Here's how the part is built. I have some questions about the finished solid (model axes, mm). Face numbers are marked on the shaded views. A direction names the side the tool comes from. Round coordinates to 2 decimals unless told otherwise and drop trailing zeros. Write each loop counter-clockwise with the first axis right and the second up, starting at its lowest first coordinate (ties: lowest second). Pieces come first, ordered by that corner, then holes. Notation, with made-up numbers: (40.25, 14) -> (57.25, 14) arc R28 ccw to (57.25, 45) -> close; hole circle Ø8 at (-3.75, 10). An arc over 180 degrees is marked (long way). Put each result on its own line as item: value. Start each with the question number.
1) Will these pins go through, and if not, where does the flat tip stop? P1, Ø1, axis at y = -4.5, z = 21.5, coming from the +X side; P2, Ø19, axis at x = -3.5, z = 16.5, coming from the +Y side; P3, Ø3.5, axis at x = -18.5, y = 18, coming from the -Z side; P4, Ø3.5, axis at y = 19, z = 92.3, coming from the -X side.
2) I want a section at B-B, the plane x = -5. List the corners of the cut face in (y, z) for me, then the cut area to 3 significant figures.
3) Which directions (+Z, -Z, +X, -X, +Y, -Y) give clear straight access to the entire face, cutting with the end or side of a thin tool? Please do the marked faces 1, 2, 3, 4 and 5.
4) If I drill on line 1 along Z through (x, y) = (-18.25, 19) (3 decimals); line 2 along Y through (x, z) = (-18, 92); line 3 along X through (y, z) = (-23, 44), over which ranges is the centre line in solid material (lowest first)? Write a range as [from, to].
5) I want a section at A-A, the plane y = -19. List the corners of the cut face in (x, z) for me (3 decimals).
6) I want a section at C-C, the plane z = 26. List the corners of the cut face in (x, y) for me, then the cut area to 3 significant figures.
7) I want a section at D-D, the plane y = -1. List the corners of the cut face in (x, z) for me.
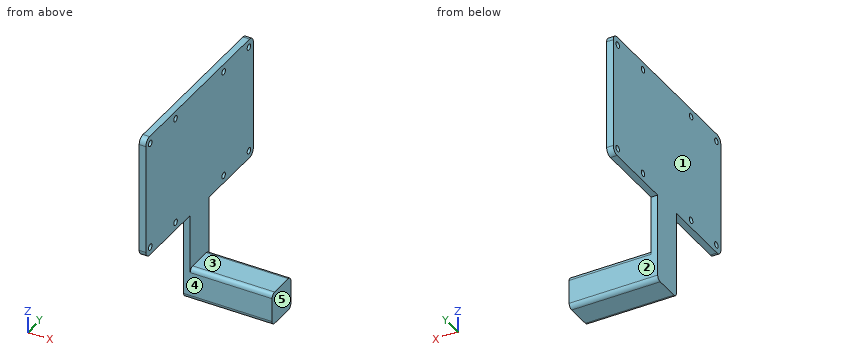
from build123d import *

# Parameters (mm, degrees)
SKETCH1_W           = 40
SKETCH1_H           = 14.8
BOSS_EXTRUDE1_DEPTH = 14.8
SKETCH3_W           = 3
SKETCH3_H           = 14.8
BOSS_EXTRUDE3_DEPTH = 25
SKETCH5_W           = 3
SKETCH5_H           = 85
BOSS_EXTRUDE4_DEPTH = 56
SKETCH6_R           = 1.375
CUT_EXTRUDE1_DEPTH  = 5
FILLET2_R           = 3
FILLET3_R           = 2


with BuildPart() as part:
    # Sketch1 → Boss-Extrude1 (new body)
    with BuildSketch(Plane.XY):
        Rectangle(SKETCH1_W, SKETCH1_H)
    extrude(amount=BOSS_EXTRUDE1_DEPTH)

    # Sketch3 → Boss-Extrude3 (add)
    with BuildSketch(Plane.XY.offset(14.8)):
        with Locations((-18.5, 0)):
            Rectangle(SKETCH3_W, SKETCH3_H)
    extrude(amount=BOSS_EXTRUDE3_DEPTH)

    # Sketch5 → Boss-Extrude4 (add)
    with BuildSketch(Plane.XY.offset(39.8)):
        with Locations((-18.5, 0)):
            Rectangle(SKETCH5_W, SKETCH5_H)
    extrude(amount=BOSS_EXTRUDE4_DEPTH)

    # Sketch6 → Cut-Extrude1 (cut)
    with BuildSketch(Plane(origin=(-17, 0, 0), x_dir=(0, 0, -1), z_dir=(1, 0, 0))):
        with Locations((-92.3, 39)):
            Circle(SKETCH6_R)
        with Locations((-43.3, 39)):
            Circle(SKETCH6_R)
        with Locations((-43.3, -19)):
            Circle(SKETCH6_R)
        with Locations((-92.3, -19)):
            Circle(SKETCH6_R)
    cut_extrude1 = extrude(amount=-CUT_EXTRUDE1_DEPTH, mode=Mode.SUBTRACT)

    # Fillet2
    fillet2_edges = [part.edges().sort_by_distance(p)[0] for p in [
        (-18.5, -42.5, 39.8),
        (-18.5, 42.5, 39.8),
        (-18.5, -42.5, 95.8),
        (-18.5, 42.5, 95.8),
    ]]
    fillet(fillet2_edges, radius=FILLET2_R)

    # Mirror1: Cut-Extrude1 across plane
    add(cut_extrude1.mirror(Plane.ZX), mode=Mode.SUBTRACT)

    # Fillet3
    fillet3_edges = [part.edges().sort_by_distance(p)[0] for p in [
        (1.5, 7.4, 14.8),
        (1.5, -7.4, 14.8),
        (0, 7.4, 0),
        (0, -7.4, 0),
    ]]
    fillet(fillet3_edges, radius=FILLET3_R)


solid = part.part
Findings:
1. P1: stops at x = -17
1. P2: stops at y = 7.4
1. P3: stops at z = 39.8
1. P4: stops at x = -20
2. outline: (-7.4, 2) arc R2 ccw to (-5.4, 0) -> (5.4, 0) arc R2 ccw to (7.4, 2) -> (7.4, 12.8) arc R2 ccw to (5.4, 14.8) -> (-5.4, 14.8) arc R2 ccw to (-7.4, 12.8) -> close
2. area: 216 mm2
3. face 1: +Z, -Z, -X, +Y, -Y
3. face 2: -Z, +X, -X, +Y
3. face 3: +Z, +X, +Y, -Y
3. face 4: -Z, +X, -X, -Y
3. face 5: +Z, -Z, +X, +Y, -Y
4. line 1: z = [39.8, 41.925], [44.675, 90.925], [93.675, 95.8]
4. line 2: y = [-42.5, -40.34], [-37.66, -20.34], [-17.66, 17.66], [20.34, 37.66], [40.34, 42.5]
4. line 3: x = [-20, -17]
5. outline: (-20, 39.8) -> (-17, 39.8) -> (-17, 41.925) -> (-20, 41.925) -> close; (-20, 44.675) -> (-17, 44.675) -> (-17, 90.925) -> (-20, 90.925) -> close; (-20, 93.675) -> (-17, 93.675) -> (-17, 95.8) -> (-20, 95.8) -> close
6. outline: (-20, -7.4) -> (-17, -7.4) -> (-17, 7.4) -> (-20, 7.4) -> close
6. area: 44.4 mm2
7. outline: (-20, 0) -> (20, 0) -> (20, 14.8) -> (-17, 14.8) -> (-17, 95.8) -> (-20, 95.8) -> close
